Check sheet for the modelled part. Datum: model origin and axes. Units: mm. Face numbers are marked on the shaded views. A direction names the side the tool comes from. Round coordinates to 2 decimals unless told otherwise and drop trailing zeros. Order: outer loops, then holes, each group sorted by start corner. A loop starts at its lowest first (then second) coordinate and runs counter-clockwise, first axis right, second up. Notation, with made-up numbers: M 1,59.25 L 12,59.25 A10 ccw 12,74.25 Z; hole C 89.25,68 d2. An arc over 180 degrees is marked long. One line per item, written item: value. Start each with the question number.
(1) Cross-section at D-D, the plane x = -11.5. Enter the section's corners in (y, z), and give its area (3 significant figures).
(2) Thickness scan on L1, parallel to Y at x = -17.25, z = 2; L2, parallel to Z at x = -15.5, y = 2.65; L3, parallel to Y at x = -1, z = 6.25. Record the ranges inside material, lowest first.
(3) Access from +Z, -Z, +X, -X, +Y, -Y to the whole of each face (thin tool, end or side, straight path). Record for the marked faces 1, 2 and 3.
(4) Cross-section at B-B, the plane z = 7.5. Enter the section's corners in (x, y), and give its area (3 significant figures).
(5) Depth check by flat-ended pin: pin 1 Ø3.5 at (x, z) = (-17, 8) entering from +Y; pin 2 Ø5.5 at (x, z) = (-6, 8) entering from +Y; pin 3 Ø1 at (x, y) = (-3, 6.5) entering from -Z; pin 4 Ø3 at (y, z) = (7.5, 7.5) entering from -X. Enter the tip coordinate at first touch or a pass-through.
(6) Cross-section at C-C, the plane y = 3.25. Enter the section's corners in (x, z).
(7) Release check for a two-part mould opening along X. For the marked faces 4, 5, 6 and 7 record: released by +X, released by -X, zero draft, split by the parting line, or undercut.
(8) Cross-section at A-A, the plane x = -15.5. Enter the section's corners in (y, z).
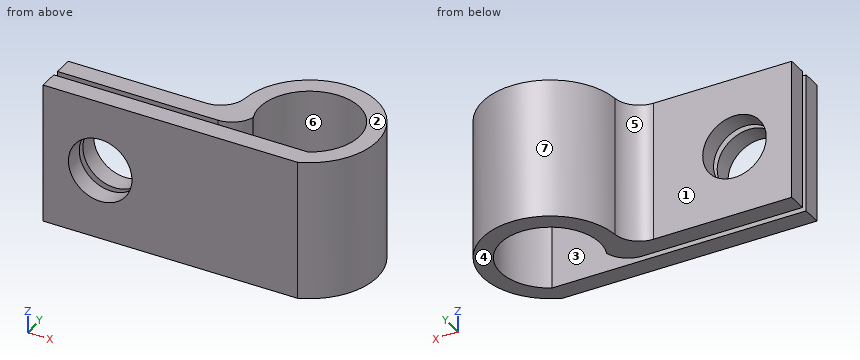
from build123d import *

# Parameters (mm, degrees)
SKETCH1_W           = 14.546192004
SKETCH1_H           = 1.5
SKETCH1_W_2         = 20
BOSS_EXTRUDE1_DEPTH = 11
SKETCH2_R           = 2.5
CUT_EXTRUDE1_DEPTH  = 26.026570584
FILLET1_R           = 2
FILLET2_R           = 2


with BuildPart() as part:
    # Sketch1 → Boss-Extrude1 (new body)
    with BuildSketch(Plane.XY):
        with Locations((-12.726903998, 2.75)):
            Rectangle(SKETCH1_W, SKETCH1_H)
        with BuildLine():
            Line((0, 1.5), (0, 0))
            ThreePointArc((0, 0), (0.523071842, 9.697161138), (-6.953807996, 3.5))
            Line((-6.953807996, 3.5), (-5.453807996, 3.5))
            ThreePointArc((-5.453807996, 3.5), (-0.488055957, 8.605123673), (0, 1.5))
        make_face()
        with Locations((-10, 0.75)):
            Rectangle(SKETCH1_W_2, SKETCH1_H)
    extrude(amount=BOSS_EXTRUDE1_DEPTH)

    # Sketch2 → Cut-Extrude1 (cut, through all)
    with BuildSketch(Plane(origin=(0, 0, 0), x_dir=(-1, 0, 0), z_dir=(0, -1, 0))):
        with Locations(Location((15.5, -5.5, 0), (0, 0, 270))):
            Circle(SKETCH2_R)
    extrude(amount=-CUT_EXTRUDE1_DEPTH, mode=Mode.SUBTRACT)

    # Fillet1
    fillet1_edges = [part.edges().sort_by_distance(p)[0] for p in [
        (-6.953807996, 3.5, 5.5),
    ]]
    fillet(fillet1_edges, radius=FILLET1_R)

    # Fillet2
    # the kernel refuses this fillet: 2 mm, written as the material it takes off along each edge
    with BuildSketch(Plane(origin=(-5.453807996, 2, -4.841229183), x_dir=(-1, 0, 0), z_dir=(0, 0, 1))) as fillet2_piece_1:
        with BuildLine():
            CenterArc((1.936491673, -2), FILLET2_R, 90, 75.522487814)
            Line((0, -1.5), (-0.038729833, -1.49))
            ThreePointArc((-0.038729833, -1.49), (-0.04, -0.75), (-0.04, 0))
            Line((-0.04, 0), (0, 0.04))
            Line((0, 0.04), (1.936491673, 0.04))
            Line((1.936491673, 0.04), (1.936491673, 0))
        make_face()
    extrude(amount=20.682458366, mode=Mode.SUBTRACT)


solid = part.part
Values found:
1. outline: M 0,0 L 1.5,0 L 1.5,11 L 0,11 Z; M 2,0 L 3.5,0 L 3.5,11 L 2,11 Z
1. area: 33.0 mm^2
2. L1: 0 to 1.5, 2 to 3.5
2. L2: 0 to 3, 8 to 11
2. L3: 0 to 1.5, 8.75 to 10.19
3. face 1: +Z, -Z, -X, +Y
3. face 2: +Z, +X, -X, +Y, -Y
3. face 3: +Z, -Z, -X
4. outline: M -20,0 L -17,0 L -17,1.5 L -20,1.5 Z; M -20,2 L -17,2 L -17,3.5 L -20,3.5 Z; M -14,0 L 0,0 A5.3 ccw long -7.15,5.35 A2 cw -9.14,3.5 L -14,3.5 L -14,2 L -7.39,2 A2 ccw -5.45,3.5 A3.9 cw long 0,1.5 L -14,1.5 Z
4. area: 72.8 mm^2
5. pin 1: y = 3.5
5. pin 2: y = 10.08
5. pin 3: through
5. pin 4: x = -7.06
6. outline: M -20,0 L -5.54,0 L -5.54,11 L -20,11 Z; M 1.68,0 L 3.16,0 L 3.16,11 L 1.68,11 Z; hole C -15.5,5.5 d5
7. face 4: zero draft
7. face 5: released by -X
7. face 6: undercut
7. face 7: split by the parting line
8. outline: M 0,0 L 1.5,0 L 1.5,3 L 0,3 Z; M 0,8 L 1.5,8 L 1.5,11 L 0,11 Z; M 2,0 L 3.5,0 L 3.5,3 L 2,3 Z; M 2,8 L 3.5,8 L 3.5,11 L 2,11 Z
